```python
from build123d import *

# Parameters (mm, degrees)
CYLINDER1799_R              = 3
CYLINDER1799_DEPTH          = 20
CYLINDER1788_R              = 1
CYLINDER1788_DEPTH          = 20
CYLINDER1789_R              = 1
CYLINDER1789_DEPTH          = 20
COMPOUND878_PLACEMENT_ANGLE = 90
CYLINDER1941_R              = 7
CYLINDER1941_DEPTH          = 13


with BuildPart() as obj1:
    # Cylinder1799 → Cylinder1799 (new body)
    with BuildSketch(Plane.XY.offset(69)):
        Circle(CYLINDER1799_R)
    extrude(amount=CYLINDER1799_DEPTH)


with BuildPart() as obj2:
    # Cylinder1788 → Cylinder1788 (new body)
    with BuildSketch(Plane(origin=(-3.5, -3.5, 0), x_dir=(1, 0, 0), z_dir=(0, 0, 1))):
        Circle(CYLINDER1788_R)
    extrude(amount=CYLINDER1788_DEPTH)


with BuildPart() as compound878:
    # Cylinder1789 → Cylinder1789 (new body)
    with BuildSketch(Plane(origin=(3.5, 3.5, 0), x_dir=(1, 0, 0), z_dir=(0, 0, 1))):
        Circle(CYLINDER1789_R)
    extrude(amount=CYLINDER1789_DEPTH)

    # Compound878: union obj2
    add(obj2.part)


with BuildPart() as compound878_1:
    # Compound878 placement: moved
    add(compound878.part.moved(Location((0, 0, 78))).rotate(Axis((0, 0, 78), (0, 0, 1)), COMPOUND878_PLACEMENT_ANGLE))


with BuildPart() as cut667:
    # Cylinder1941 → Cylinder1941 (new body)
    with BuildSketch(Plane.XY.offset(-27.5)):
        Circle(CYLINDER1941_R)
    extrude(amount=CYLINDER1941_DEPTH)


with BuildPart() as cut667_1:
    # Compound876 placement: moved
    add(cut667.part.moved(Location((0, 0, 107))))

    # Cut714: cut Compound878
    add(compound878_1.part, mode=Mode.SUBTRACT)

    # Cut667: cut obj1
    add(obj1.part, mode=Mode.SUBTRACT)


solid = cut667_1.part
```
Design review of the part built by this model. Coordinates are the model's own, in mm. A direction names the side the tool comes from. Coordinates: 2 decimals unless noted, no trailing zeros. Order: outer loops, then holes, each group sorted by start corner. A loop starts at its lowest first (then second) coordinate and runs counter-clockwise, first axis right, second up. Notation, with made-up numbers: (-1, 49) - (10, 49) arc R13 cw to (10, 68) - close; hole circle Ø3 at (-29.5, -32). An arc over 180 degrees is marked (long way). One line per question, with ' | ' between items.
Q1. For faces 1 (the cylindrical face through (-3, 0, 84)), 2 (the flat face through (1, -3, 79.5)), list the 3-axis set-ups (+Z, -Z, +X, -X, +Y, -Y) from which the entire face can be reached by the end or side of a thin tool; tool diameter is ignored.
Answer key:
face 1: -Z | face 2: -Z, +X, -X, +Y, -Y
Q2. Consider section B-B, the plane y = -3.25. Give the boundary of the cut face in (x, z).
Answer key:
outline: (-6.2, 79.5) - (2.53, 79.5) - (2.53, 92.5) - (-6.2, 92.5) - close; (4.47, 79.5) - (6.2, 79.5) - (6.2, 92.5) - (4.47, 92.5) - close
Q3. Consider section C-C, the plane z = 88. Give the boundary of the cut face in (x, y).
Answer key:
outline: circle Ø14 at (0, 0); hole circle Ø2 at (-3.5, 3.5); hole circle Ø6 at (0, 0); hole circle Ø2 at (3.5, -3.5)
Q4. Clearance check with flat-ended pins moving along their axes: pin 1 Ø2.5 at (x, y) = (-3.5, 3.5) entering from +Z; pin 2 Ø5 at (x, y) = (0, 0) entering from -Z; pin 3 Ø3 at (x, z) = (-2.5, 88.5) entering from +Y; pin 4 Ø3 at (x, z) = (4, 90.5) entering from +Y. State where each tip first meets the part, or that it passes through.
Answer key:
pin 1: stops at z = 92.5 | pin 2: stops at z = 89 | pin 3: stops at y = 6.93 | pin 4: stops at y = 6.54
Q5. Consider section D-D, the plane x = 2. Give the boundary of the cut face in (y, z).
Answer key:
outline: (-6.71, 79.5) - (-2.24, 79.5) - (-2.24, 89) - (2.24, 89) - (2.24, 79.5) - (6.71, 79.5) - (6.71, 92.5) - (-6.71, 92.5) - close
Q6. The part is to be moulded in two halves that separate along X. For faces 3 (the cylindrical face through (6.466, -2.681, 85.909)), 4 (the cylindrical face through (3.5, -4.5, 85.9)), 5 (the flat face through (0, 0, 92.5)), say which applies: +X half, -X half, draft (parallel to the pull), parting line (faces both ways), or undercut.
Answer key:
face 3: parting line | face 4: undercut | face 5: draft
Q7. To check wall thickness, follow line 1 along Y through (x, z) = (0, 82); line 2 along Z through (x, y) = (0.5, -2.5); line 3 along X through (y, z) = (3.5, 82.5). State the ranges of each line that lie inside material, in increasing order.
Answer key:
line 1: y = -7 to -3, 3 to 7 | line 2: z = 89 to 92.5 | line 3: x = -6.06 to -4.5, -2.5 to 6.06
Q8. Consider section A-A, the plane x = -2.75. Give the boundary of the cut face in (y, z).
Answer key:
outline: (-6.44, 79.5) - (-1.2, 79.5) - (-1.2, 89) - (1.2, 89) - (1.2, 79.5) - (2.84, 79.5) - (2.84, 92.5) - (-6.44, 92.5) - close; (4.16, 79.5) - (6.44, 79.5) - (6.44, 92.5) - (4.16, 92.5) - close
